Can you work these out from the model? Positions are in its coordinate system, mm. Round coordinates to 2 decimals unless told otherwise and drop trailing zeros. Write each loop counter-clockwise with the first axis right and the second up, starting at its lowest first coordinate (ties: lowest second). Pieces come first, ordered by that corner, then holes. Notation, with made-up numbers: M 67,41.5 L 87,41.5 A25 cw 87,72.5 Z; hole C -37.75,19 d6. An arc over 180 degrees is marked long. Answer as a JSON object with one key per item and string values. Group by question number.
1) Suppose I cut it at A-A, the plane z = 112. Write out the boundary of the cut face in (x, y), and give its area (3 significant figures).
2) Please list where these lines run through material, in increasing order: L1, parallel to X at y = -3, z = 200; L2, parallel to X at y = 6.5, z = 346.5; L3, parallel to Y at x = -25, z = 203. Write a range as [from, to].
3) Suppose I cut it at B-B, the plane x = 9.5. Write out the boundary of the cut face in (y, z).
4) I'm going to push flat-ended pins straight in: pin 1 Ø8 at (x, y) = (-25, -2.5) entering from +Z; pin 2 Ø13.5 at (x, z) = (-9, 168.5) entering from +Y. Where does each tip first touch, or does it pass through?
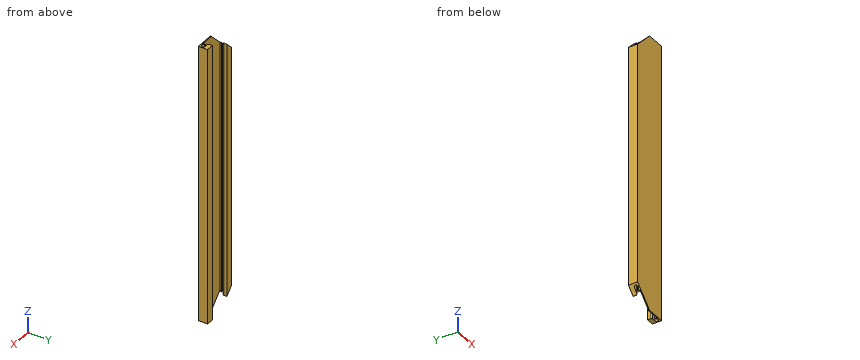
from build123d import *

# Parameters (mm, degrees)
SKETCH_1_W               = 60
SKETCH_1_H               = 15
EXTRUDE_1_DEPTH          = 510
SKETCH_2_R               = 3
CUT_EXTRUDE_1_DEPTH      = 511.936639908
CUT_EXTRUDE_2_DEPTH      = 511.936639908
SKETCH_4_W               = 36.3
SKETCH_4_H               = 7
CUT_EXTRUDE_3_DEPTH      = 511.936639908
FILLET_1_R               = 2
CUT_EXTRUDE_4_DEPTH      = 512.101751122
CUT_EXTRUDE_6_DEPTH      = 512.101751122
CUT_EXTRUDE_6_DEPTH_BACK = 512.101751122
SKETCH_7_W               = 30
SKETCH_7_H               = 30


with BuildPart() as part:
    # 스케치1 → 보스-돌출1 (new body)
    with BuildSketch(Plane.XY):
        Rectangle(SKETCH_1_W, SKETCH_1_H)
    extrude(amount=EXTRUDE_1_DEPTH)

    # 스케치2 → 컷-돌출1 (cut, through all)
    with BuildSketch(Plane(origin=(0, 0, 0), x_dir=(-1, 0, 0), z_dir=(0, 0, -1))):
        with Locations((-25, -2.5)):
            Circle(SKETCH_2_R)
        with Locations((25, -2.5)):
            Circle(SKETCH_2_R)
    extrude(amount=-CUT_EXTRUDE_1_DEPTH, mode=Mode.SUBTRACT)

    # 스케치3 → 컷-돌출2 (cut, through all)
    with BuildSketch(Plane(origin=(0, 0, 0), x_dir=(-1, 0, 0), z_dir=(0, 0, -1))):
        with BuildLine():
            Line((-22.171572875, -6), (22.171572875, -6))
            ThreePointArc((22.171572875, -6), (20.939339828, -4.439339828), (20.5, -2.5))
            Line((20.5, -2.5), (25, -2.5))
            Line((25, -2.5), (25, 0.5))
            Line((25, 0.5), (-25, 0.5))
            Line((-25, 0.5), (-25, -2.5))
            Line((-25, -2.5), (-20.5, -2.5))
            ThreePointArc((-20.5, -2.5), (-20.939339828, -4.439339828), (-22.171572875, -6))
        make_face()
    extrude(amount=-CUT_EXTRUDE_2_DEPTH, mode=Mode.SUBTRACT)

    # 스케치4 → 컷-돌출3 (cut, through all)
    with BuildSketch(Plane(origin=(0, 0, 0), x_dir=(-1, 0, 0), z_dir=(0, 0, -1))):
        with Locations((0.006888359, 4)):
            Rectangle(SKETCH_4_W, SKETCH_4_H)
    extrude(amount=-CUT_EXTRUDE_3_DEPTH, mode=Mode.SUBTRACT)

    # 필렛1
    fillet_1_edges = [part.edges().sort_by_distance(p)[0] for p in [
        (-18.156888359, 0.5, 255),
        (18.143111641, 0.5, 255),
    ]]
    fillet(fillet_1_edges, radius=FILLET_1_R)

    # 스케치5 → 컷-돌출4 (cut, through all)
    with BuildSketch(Plane.XZ.offset(7.5)):
        Polygon((-30, 510), (-30, 450), (30, 510), align=None)
        Polygon((-30, 0), (30, 0), (-30, 60), align=None)
    extrude(amount=-CUT_EXTRUDE_4_DEPTH, mode=Mode.SUBTRACT)

    # 스케치7 → 컷-돌출6 (cut, two sides: drawn at the far end of the back side and taken through both)
    with BuildSketch(Plane.XZ.offset(7.5).offset(-CUT_EXTRUDE_6_DEPTH_BACK)):
        with Locations((15, 15)):
            Rectangle(SKETCH_7_W, SKETCH_7_H)
        with Locations((15, 495)):
            Rectangle(SKETCH_7_W, SKETCH_7_H)
    extrude(amount=CUT_EXTRUDE_6_DEPTH + CUT_EXTRUDE_6_DEPTH_BACK, mode=Mode.SUBTRACT)


solid = part.part
Results:
{
 "1": {"outline": "M -30,-7.5 L 30,-7.5 L 30,7.5 L 18.14,7.5 L 18.14,2.5 A2 ccw 20.14,0.5 L 25,0.5 A3 cw long 22,-2.5 L 20.5,-2.5 A4.5 ccw 22.17,-6 L -22.17,-6 A4.5 ccw -20.5,-2.5 L -22,-2.5 A3 cw long -25,0.5 L -20.16,0.5 A2 ccw -18.16,2.5 L -18.16,7.5 L -30,7.5 Z", "area": "305 mm^2"},
 "2": {"L1": "[-30, -27.96], [-22.04, -20.53], [20.53, 22.04], [27.96, 30]", "L2": "[-30, -18.16], [18.14, 30]", "L3": "[-7.5, -5.5], [0.5, 7.5]"},
 "3": {"outline": "M -7.5,30 L -6,30 L -6,480 L -7.5,480 Z"},
 "4": {"pin 1": "z = 459", "pin 2": "y = -6"}
}
